Source: CAD feature listing. Evaluate the final solid. Frame: model axes, mm. Face numbers are marked on the shaded views. A direction names the side the tool comes from. Give positions to 0.01 mm unless a question says otherwise; leave off trailing zeros. Order: outer loops, then holes, each group sorted by start corner. A loop starts at its lowest first (then second) coordinate and runs counter-clockwise, first axis right, second up.
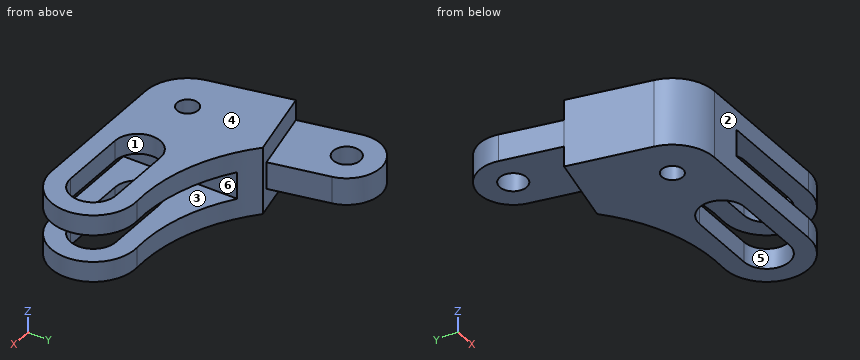
from build123d import *

# Parameters (mm, degrees)
SKETCH2_R               = 6.25
BOSS_EXTRUDE1_DEPTH     = 20
CUT_EXTRUDE1_DEPTH      = 123.932823709
CUT_EXTRUDE1_DEPTH_BACK = 123.932823709
SKETCH4_W               = 90
SKETCH4_H               = 16
SKETCH5_R               = 8
BOSS_EXTRUDE2_DEPTH     = 8


with BuildPart() as part:
    # Sketch2 → Boss-Extrude1 (new, symmetric)
    with BuildSketch(Plane.XY):
        with BuildLine():
            Line((0, -25), (85, -25))
            ThreePointArc((85, -25), (109.987866766, 0.7787904), (83.443175141, 24.951478841))
            ThreePointArc((83.443175141, 24.951478841), (43.835315137, 30.493200705), (9.566653282, 51.11241674))
            Line((9.566653282, 51.11241674), (-34.446959185, 41.742148997))
            Line((-34.446959185, 41.742148997), (-24.452006926, -5.205704301))
            ThreePointArc((-24.452006926, -5.205704301), (-15.729866377, -19.43119409), (0, -25))
        make_face()
        Circle(SKETCH2_R, mode=Mode.SUBTRACT)
        with BuildLine():
            Line((85, -13.5), (45, -13.5))
            ThreePointArc((45, -13.5), (31.5, 0), (45, 13.5))
            Line((45, 13.5), (85, 13.5))
            ThreePointArc((85, 13.5), (98.5, 0), (85, -13.5))
        make_face(mode=Mode.SUBTRACT)
    extrude(amount=BOSS_EXTRUDE1_DEPTH, both=True)

    # Sketch4 → Cut-Extrude1 (cut, two sides: drawn at the far end of the back side and taken through both)
    with BuildSketch(Plane(origin=(0, 0, 0), x_dir=(1, 0, 0), z_dir=(0, 1, 0)).offset(-CUT_EXTRUDE1_DEPTH_BACK)):
        with Locations((65, 0)):
            Rectangle(SKETCH4_W, SKETCH4_H)
    extrude(amount=CUT_EXTRUDE1_DEPTH + CUT_EXTRUDE1_DEPTH_BACK, mode=Mode.SUBTRACT)

    # Sketch5 → Boss-Extrude2 (add, symmetric)
    with BuildSketch(Plane.XY):
        with BuildLine():
            Line((-34.446959185, 41.742148997), (-41.734945207, 75.974958694))
            ThreePointArc((-41.734945207, 75.974958694), (-26.337903107, 99.701127676), (-2.611734125, 84.304085576))
            Line((-2.611734125, 84.304085576), (4.676251897, 50.071275879))
            Line((4.676251897, 50.071275879), (-34.446959185, 41.742148997))
        make_face()
        with Locations((-22.173339666, 80.139522135)):
            Circle(SKETCH5_R, mode=Mode.SUBTRACT)
    extrude(amount=BOSS_EXTRUDE2_DEPTH, both=True)


solid = part.part
1) Ray query, L1, parallel to Z at x = 30, y = -8; L2, parallel to Z at x = -14, y = 49; L3, parallel to Y at x = 55.5, z = -16. Return the intervals inside material, ascending.
Checks:
L1: z = -20 to -8, 8 to 20
L2: z = -8 to 8
L3: y = -25 to -13.5, 13.5 to 27.14
2) Section query B-B on y = 0. Output: boundary loops of the cut face in (x, z), and give its area (3 significant figures).
Checks:
outline: (-25.56, -20) - (-6.25, -20) - (-6.25, 20) - (-25.56, 20) - close; (6.25, -20) - (31.5, -20) - (31.5, -8) - (20, -8) - (20, 8) - (31.5, 8) - (31.5, 20) - (6.25, 20) - close; (98.5, -20) - (110, -20) - (110, -8) - (98.5, -8) - close; (98.5, 8) - (110, 8) - (110, 20) - (98.5, 20) - close
area: 1,870 mm2
3) Pull-direction query (X, two-part tool) for the marked faces 4, 5 and 6; classes: +X half, -X half, draft (parallel to the pull), parting line (faces both ways), or undercut.
Checks:
face 4: draft
face 5: undercut
face 6: +X half
4) Section query D-D on y = 86.5. Output: boundary loops of the cut face in (x, z) (3 decimals).
Checks:
outline: (-41.135, -8) - (-27.026, -8) - (-27.026, 8) - (-41.135, 8) - close; (-17.321, -8) - (-3.212, -8) - (-3.212, 8) - (-17.321, 8) - close
5) First-contact query: pin 1 Ø5 at (y, z) = (9.5, -0.5) entering from +X; pin 2 Ø12 at (x, z) = (67, 10.5) entering from +Y; pin 3 Ø10 at (y, z) = (17, 11.5) entering from +X. Flat tips, straight axial feed; report the tip coordinate or a pass-through.
Checks:
pin 1: stops at x = 20
pin 2: stops at y = 26.08
pin 3: stops at x = 106.93
6) Section query A-A on x = -21. Output: boundary loops of the cut face in (y, z).
Checks:
outline: (-13.56, -20) - (44.6, -20) - (44.6, -8) - (72.23, -8) - (72.23, 8) - (44.6, 8) - (44.6, 20) - (-13.56, 20) - close; (88.05, -8) - (100.11, -8) - (100.11, 8) - (88.05, 8) - close
7) Section query C-C on z = 11.5. Output: boundary loops of the cut face in (x, y).
Checks:
outline: (-34.45, 41.74) - (-24.45, -5.21) arc R25 ccw to (0, -25) - (85, -25) arc R25 ccw (long way) to (83.44, 24.95) arc R100 cw to (9.57, 51.11) - close; hole circle Ø12.5 at (0, 0); hole (45, -13.5) - (85, -13.5) arc R13.5 ccw to (85, 13.5) - (45, 13.5) arc R13.5 ccw to start
8) Reachability of the marked faces 1, 2 and 3 from +Z, -Z, +X, -X, +Y, -Y: full face, straight path, thin tool, end or side. Return the list, or none.
Checks:
face 1: +Z, -Z
face 2: +Z, -Z, +X, -X, -Y
face 3: +X, +Y, -Y
